```python
from build123d import *

# Parameters (mm, degrees)
EXTRUDE_1_DEPTH     = 5
EXTRUDE_2_DEPTH     = 5
SKETCH_4_W          = 5
SKETCH_4_H          = 5
EXTRUDE_4_DEPTH     = 50
EXTRUDE_13_DEPTH    = 5
SKETCH_8_R          = 1.5
SKETCH_8_R_2        = 1.4
CUT_EXTRUDE_1_DEPTH = 87.602540378
SKETCH_9_R          = 1.5
CUT_EXTRUDE_2_DEPTH = 87.602540378
SKETCH_10_R         = 1.5
CUT_EXTRUDE_3_DEPTH = 87.602540378


with BuildPart() as part:
    # Sketch 1 → Extrude 1 (new body)
    with BuildSketch(Plane.XY):
        Polygon((0, 50), (50, 0), (50, -5), (-5, -5), (-5, 50), align=None)
    extrude(amount=EXTRUDE_1_DEPTH)



with BuildPart() as body_2:
    # Sketch 2 → Extrude 2 (new body)
    with BuildSketch(Plane(origin=(0, 0, 0), x_dir=(0, 0, -1), z_dir=(1, 0, 0))):
        Polygon((0, 0), (50, 0), (0, 50), align=None)
    extrude(amount=-EXTRUDE_2_DEPTH)

    # Sketch 4 → Extrude 4 (add)
    with BuildSketch(Plane.XY):
        with Locations((-2.5, -2.5)):
            Rectangle(SKETCH_4_W, SKETCH_4_H)
    extrude(amount=-EXTRUDE_4_DEPTH)


with BuildPart() as part_1:
    add(part.part)

    add(body_2.part)  # Extrude 13 merges body 2
    # Sketch 7 → Extrude 13 (add)
    with BuildSketch(Plane.XZ.offset(5)):
        Polygon((50, 0), (0, 0), (0, -50), align=None)
    extrude(amount=-EXTRUDE_13_DEPTH)

    # Sketch 8 → Cut-Extrude 1 (cut, through all)
    with BuildSketch(Plane(origin=(0, 0, 0), x_dir=(0, 0, -1), z_dir=(1, 0, 0))):
        with Locations((5, 30)):
            Circle(SKETCH_8_R)
        with Locations((5, 5)):
            Circle(SKETCH_8_R_2)
        with Locations((30, 5)):
            Circle(SKETCH_8_R)
    extrude(amount=-CUT_EXTRUDE_1_DEPTH, mode=Mode.SUBTRACT)

    # Sketch 9 → Cut-Extrude 2 (cut, through all)
    with BuildSketch(Plane(origin=(0, 0, 0), x_dir=(-1, 0, 0), z_dir=(0, 0, -1))):
        with Locations((-5, 30)):
            Circle(SKETCH_9_R)
        with Locations((-5, 5)):
            Circle(SKETCH_9_R)
        with Locations((-30, 5)):
            Circle(SKETCH_9_R)
    extrude(amount=-CUT_EXTRUDE_2_DEPTH, mode=Mode.SUBTRACT)

    # Sketch 10 → Cut-Extrude 3 (cut, through all)
    with BuildSketch(Plane(origin=(0, 0, 0), x_dir=(1, 0, 0), z_dir=(0, 1, 0))):
        with Locations(Location((5, 30, 0), (0, 0, 270))):
            Circle(SKETCH_10_R)
        with Locations(Location((5, 5, 0), (0, 0, 270))):
            Circle(SKETCH_10_R)
        with Locations(Location((30, 5, 0), (0, 0, 270))):
            Circle(SKETCH_10_R)
    extrude(amount=-CUT_EXTRUDE_3_DEPTH, mode=Mode.SUBTRACT)


solid = part_1.part
```
Design review of the part built by this model. Coordinates are the model's own, in mm. A direction names the side the tool comes from. Coordinates: 2 decimals unless noted, no trailing zeros. Order: outer loops, then holes, each group sorted by start corner. A loop starts at its lowest first (then second) coordinate and runs counter-clockwise, first axis right, second up.
1) Clearance check with flat-ended pins moving along their axes: pin 1 (25 mm diameter, centred on x = 28.5, z = -13.5, fed in from +Y); pin 2 (3.5 mm diameter, centred on x = 30, y = 5, fed in from -Z); pin 3 (10 mm diameter, centred on y = 16, z = -7.5, fed in from +X). State where each tip first meets the part, or that it passes through.
2) Wall thickness on line 1 along X through (y, z) = (-2.85, -5); line 2 along Y through (x, z) = (23, -5); line 3 along Y through (x, z) = (-2, -5): over which ranges is each line inside the solid? List them lowest first.
3) Mouldability with a two-part tool opening along X and no side actions: class faces 3 (the flat face through (19, 0, -19)), 4 (the flat face through (25, 25, 2)), 5 (the cylindrical face through (6.2, 4.1, 2.5)) as +X half, -X half, draft (parallel to the pull), parting line (faces both ways), or undercut.
4) Take a section at C-C, the plane x = 5. Give the boundary of the cut face in (y, z).
5) Take a section at A-A, the plane z = -5. Give the boundary of the cut face in (x, y), and give its area (3 significant figures).
6) For faces 1 (the flat face through (14, 14, 0)), 2 (the flat face through (-3, 50, 2)), list the 3-axis set-ups (+Z, -Z, +X, -X, +Y, -Y) from which the entire face can be reached by the end or side of a thin tool; tool diameter is ignored.
7) Take a section at B-B, the plane z = -30. Give the boundary of the cut face in (x, y).
8) Take a section at D-D, the plane y = 30. Give the boundary of the cut face in (x, z).
Returned:
1. pin 1: stops at y = 0
1. pin 2: stops at z = 0
1. pin 3: stops at x = 0
2. line 1: x = -5 to 3.5, 6.5 to 28.5, 31.5 to 45
2. line 2: y = -5 to 0
2. line 3: y = -5 to 3.6, 6.4 to 28.5, 31.5 to 45
3. face 3: draft
3. face 4: +X half
3. face 5: undercut
4. outline: (-5, -45) - (0, -45) - (0, -31.5) - (-5, -31.5) - close; (-5, -28.5) - (0, -28.5) - (0, -6.5) - (-5, -6.5) - close; (-5, -3.5) - (0, -3.5) - (0, 0) - (3.5, 0) - (3.5, 5) - (-5, 5) - close; (6.5, 0) - (28.5, 0) - (28.5, 5) - (6.5, 5) - close; (31.5, 0) - (45, 0) - (45, 5) - (31.5, 5) - close
5. outline: (-5, -5) - (3.5, -5) - (3.5, 0) - (0, 0) - (0, 3.6) - (-5, 3.6) - close; (-5, 6.4) - (0, 6.4) - (0, 28.5) - (-5, 28.5) - close; (-5, 31.5) - (0, 31.5) - (0, 45) - (-5, 45) - close; (6.5, -5) - (28.5, -5) - (28.5, 0) - (6.5, 0) - close; (31.5, -5) - (45, -5) - (45, 0) - (31.5, 0) - close
5. area: 416 mm2
6. face 1: -Z, +X, +Y
6. face 2: +Z, -Z, +X, -X, +Y
7. outline: (-5, -5) - (3.5, -5) - (3.5, 0) - (0, 0) - (0, 3.5) - (-5, 3.5) - close; (-5, 6.5) - (0, 6.5) - (0, 20) - (-5, 20) - close; (6.5, -5) - (20, -5) - (20, 0) - (6.5, 0) - close
8. outline: (-5, -20) - (0, -20) - (0, -6.5) - (-5, -6.5) - close; (-5, -3.5) - (0, -3.5) - (0, 0) - (3.5, 0) - (3.5, 5) - (-5, 5) - close; (6.5, 0) - (20, 0) - (20, 5) - (6.5, 5) - close
